The figure shows three views and two pictorial views of one solid part (mm, origin at its lowest corner). Answer the questions. Coordinates: 2 decimals unless noted, no trailing zeros. Loops run counter-clockwise (first coordinate to the right, second up) from the corner with the lowest first, then second, coordinate; pieces in that order, holes last. Notation, with made-up numbers: (21, -25) -> (68, -25) arc R30 cw to (68, -3) -> close; hole circle Ø8 at (-31.75, 26.5). An arc over 180 degrees is marked (long way). Answer in a Markdown table with one row per item.
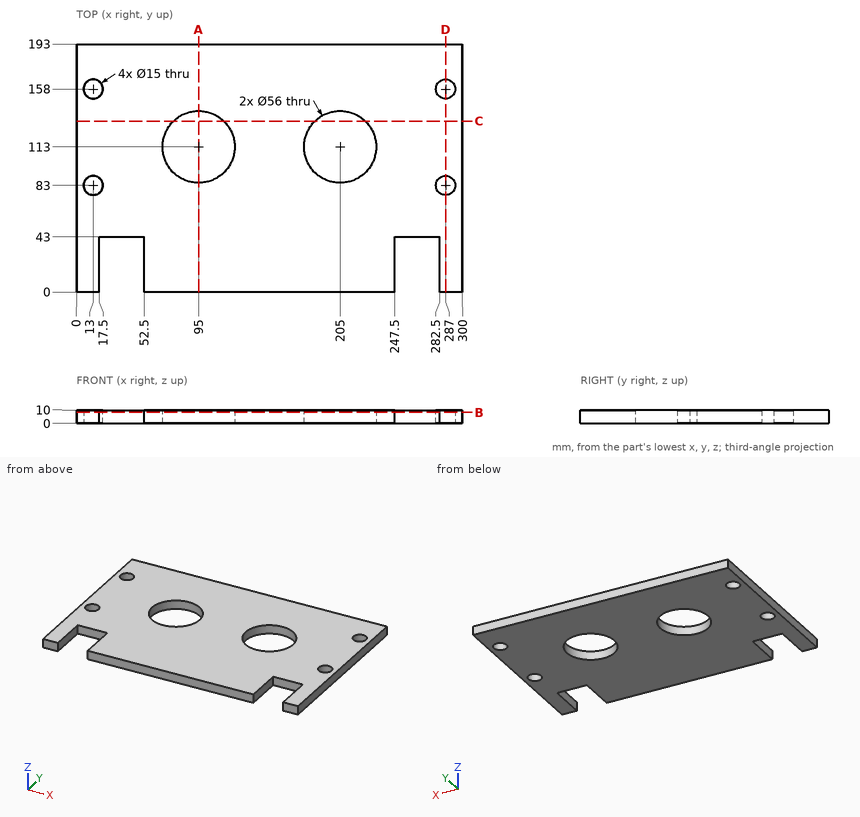
Item 1: A cutting plane is placed at D-D, the plane x = 287. Determine the outline of the cut face in (y, z).
Findings below:
| item | result |
|---|---|
| outline | (0, 0) -> (75.5, 0) -> (75.5, 10) -> (0, 10) -> close; (90.5, 0) -> (150.5, 0) -> (150.5, 10) -> (90.5, 10) -> close; (165.5, 0) -> (193, 0) -> (193, 10) -> (165.5, 10) -> close |
Item 2: A cutting plane is placed at A-A, the plane x = 95. Determine the outline of the cut face in (y, z), plus the area to 3 significant figures.
Findings below:
| item | result |
|---|---|
| outline | (0, 0) -> (85, 0) -> (85, 10) -> (0, 10) -> close; (141, 0) -> (193, 0) -> (193, 10) -> (141, 10) -> close |
| area | 1,370 mm2 |
Item 3: A cutting plane is placed at B-B, the plane z = 8.25. Determine the outline of the cut face in (x, y), plus the area to 3 significant figures.
Findings below:
| item | result |
|---|---|
| outline | (0, 0) -> (17.5, 0) -> (17.5, 43) -> (52.5, 43) -> (52.5, 0) -> (247.5, 0) -> (247.5, 43) -> (282.5, 43) -> (282.5, 0) -> (300, 0) -> (300, 193) -> (0, 193) -> close; hole circle Ø15 at (13, 83); hole circle Ø15 at (13, 158); hole circle Ø56 at (95, 113); hole circle Ø56 at (205, 113); hole circle Ø15 at (287, 83); hole circle Ø15 at (287, 158) |
| area | 49,300 mm2 |
Item 4: A cutting plane is placed at C-C, the plane y = 133. Determine the outline of the cut face in (x, z), plus the area to 3 significant figures.
Findings below:
| item | result |
|---|---|
| outline | (0, 0) -> (75.4, 0) -> (75.4, 10) -> (0, 10) -> close; (114.6, 0) -> (185.4, 0) -> (185.4, 10) -> (114.6, 10) -> close; (224.6, 0) -> (300, 0) -> (300, 10) -> (224.6, 10) -> close |
| area | 2,220 mm2 |
Item 5: Find the intervals of material crossed by probe 1 along X at (y, z) = (39.5, 3.75); probe 2 along Y at (x, z) = (13, 4); probe 3 along Y at (x, z) = (204, 1.25), in increasing order.
Findings below:
| item | result |
|---|---|
| probe 1 | x = 0 to 17.5, 52.5 to 247.5, 282.5 to 300 |
| probe 2 | y = 0 to 75.5, 90.5 to 150.5, 165.5 to 193 |
| probe 3 | y = 0 to 85.02, 140.98 to 193 |
Item 6: Flat-ended cylindrical pins translate along their axes: pin 1 Ø12 at (x, y) = (13, 158) entering from -Z; pin 2 Ø5 at (x, z) = (263.5, 6.5) entering from -Y. Find the tip coordinate at first contact, or state that the pin passes through.
Findings below:
| item | result |
|---|---|
| pin 1 | passes through |
| pin 2 | stops at y = 43 |
